Geometry check sheet. Reference: the model listing, model coordinates, mm. A direction names the side the tool comes from. Give positions to 0.01 mm unless a question says otherwise; leave off trailing zeros. Loops run counter-clockwise (first coordinate to the right, second up) from the corner with the lowest first, then second, coordinate; pieces in that order, holes last. Notation, with made-up numbers: (83.25, 25.5) - (105.25, 25.5) arc R26 ccw to (105.25, 46.5) - close; hole circle Ø10 at (18.25, -4). An arc over 180 degrees is marked (long way). Use a Markdown table: item, result. Add a question column.
1. Draft check along Y on faces 5 (the flat face through (-2, 2, -2)), 6 (the cylindrical face through (2, -5, -53)), 7 (the flat face through (-51, -10, 31)). Enter one of: pulls with the +Y half, pulls with the -Y half, needs draft (parallel to the pull), parting line crosses it, or undercut.
2. Cross-section at A-A on z = -55. Enter the section's corners in (x, y).
3. Depth check by flat-ended pin: P1, Ø1, axis at x = -61.5, y = 3.5, coming from the -Z side; P2, Ø6, axis at x = 18.5, y = 1, coming from the +Z side; P3, Ø7.5, axis at x = 3, z = -2, coming from the +Y side; P4, Ø2, axis at x = -2.5, y = -3, coming from the -Z side. Enter the tip coordinate at first touch or a pass-through.
4. Material ranges on L1, parallel to Y at x = 2.2, z = -55; L2, parallel to X at y = -8.5, z = -63.5; L3, parallel to X at y = 6.25, z = 0, recorded low to high.
5. Cross-section at B-B on z = 0. Enter the section's corners in (x, y), and give its area (3 significant figures).
6. Cross-section at C-C on y = 5.75. Enter the section's corners in (x, z).
7. Set-up check for faces 1 (the flat face through (51.29, -4.93, 30.883)), 2 (the flat face through (-1.1, -5, -60)), 3 (the flat face through (-54.171, 1.014, 33.717)), 4 (the flat face through (50.533, -4.93, 32.755)): record each of +Z, -Z, +X, -X, +Y, -Y from which the full face is reachable in a straight line by a thin tool's end or side.
8. Cross-section at D-D on z = -20.5. Enter the section's corners in (x, y), and give its area (3 significant figures).
from build123d import *

# Parameters (mm, degrees)
BOSS_EXTRUDE1_DEPTH = 2
BOSS_EXTRUDE1_DRAFT = 45
SKETCH2_R           = 2.5
CUT_EXTRUDE1_DEPTH  = 114.154761278
SKETCH3_R           = 9
SKETCH3_R_2         = 7.5
BOSS_EXTRUDE2_DEPTH = 8
SKETCH4_W           = 2
SKETCH4_H           = 20
BOSS_EXTRUDE3_DEPTH = 10
SKETCH5_R           = 2
CUT_EXTRUDE2_DEPTH  = 10
CIRPATTERN1_COUNT   = 3
CUT_EXTRUDE3_DEPTH  = 1000


# Read off the part's stored shape, not the designer's step: Boss-Extrude1
with BuildPart() as part:
    # Boss-Extrude1 outline → Boss-Extrude1 (with draft: the straight prism first)
    with BuildSketch(Plane(origin=(0, 2, 0), x_dir=(1, 0, 0), z_dir=(0, 1, 0))):
        with BuildLine():
            ThreePointArc((-3.1, 77.938373091), (-67.549981495, 39), (-69.046611026, -36.284507794))
            Line((-69.046611026, -36.284507794), (-43.119219382, -21.315321248))
            Line((-43.119219382, -21.315321248), (-40.019219382, -26.684678752))
            Line((-40.019219382, -26.684678752), (-65.946611026, -41.653865297))
            ThreePointArc((-65.946611026, -41.653865297), (0, -78), (65.946611026, -41.653865297))
            Line((65.946611026, -41.653865297), (40.019219382, -26.684678752))
            Line((40.019219382, -26.684678752), (43.119219382, -21.315321248))
            Line((43.119219382, -21.315321248), (69.046611026, -36.284507794))
            ThreePointArc((69.046611026, -36.284507794), (67.549981495, 39), (3.1, 77.938373091))
            Line((3.1, 77.938373091), (3.1, 48))
            Line((3.1, 48), (-3.1, 48))
            Line((-3.1, 48), (-3.1, 77.938373091))
        make_face()
    extrude(amount=-BOSS_EXTRUDE1_DEPTH)
    # Boss-Extrude1: the draft: its side faces are tilted about the plane it starts from
    boss_extrude1_sides = [part.faces().sort_by_distance(p)[0] for p in [
        (67.549981495, 1, -39),
        (3.1, 1, -62.969186546),
        (0, 1, -48),
        (-3.1, 1, -62.969186546),
        (-67.549981495, 1, -39),
        (-56.082915204, 1, 28.799914521),
        (-41.569219382, 1, 24),
        (-52.982915204, 1, 34.169272025),
        (0, 1, 78),
        (52.982915204, 1, 34.169272025),
        (41.569219382, 1, 24),
        (56.082915204, 1, 28.799914521),
    ]]
    draft(boss_extrude1_sides, Plane(origin=(0, 2, 0), x_dir=(1, 0, 0), z_dir=(0, 1, 0)), BOSS_EXTRUDE1_DRAFT)

    # Sketch2 → Cut-Extrude1 (cut, through all)
    with BuildSketch(Plane(origin=(0, 2, 0), x_dir=(1, 0, 0), z_dir=(0, 1, 0))):
        with Locations(Location((0, 0, 0), (0, 0, 270))):
            Circle(SKETCH2_R)
    extrude(amount=-CUT_EXTRUDE1_DEPTH, mode=Mode.SUBTRACT)

    # Sketch3 → Boss-Extrude2 (add)
    with BuildSketch(Plane(origin=(0, 2, 0), x_dir=(1, 0, 0), z_dir=(0, 1, 0))):
        with Locations(Location((0, 0, 0), (0, 0, 270))):
            Circle(SKETCH3_R)
        with Locations(Location((0, 0, 0), (0, 0, 270))):
            Circle(SKETCH3_R_2, mode=Mode.SUBTRACT)
    extrude(amount=BOSS_EXTRUDE2_DEPTH)

    # Sketch4 → Boss-Extrude3 (add)
    with BuildSketch(Plane.XZ):
        Polygon((42.751270189, 25.952627944), (60.071778265, 35.952627944), (59.071778265, 37.684678752), (41.751270189, 27.684678752), align=None)
        Polygon((43.851270189, 24.047372056), (61.171778265, 34.047372056), (62.171778265, 32.315321248), (44.851270189, 22.315321248), align=None)
        with Locations((2.1, -60)):
            Rectangle(SKETCH4_W, SKETCH4_H)
        with Locations((-2.1, -60)):
            Rectangle(SKETCH4_W, SKETCH4_H)
        Polygon((-44.851270189, 22.315321248), (-62.171778265, 32.315321248), (-61.171778265, 34.047372056), (-43.851270189, 24.047372056), align=None)
        Polygon((-42.751270189, 25.952627944), (-60.071778265, 35.952627944), (-59.071778265, 37.684678752), (-41.751270189, 27.684678752), align=None)
    extrude(amount=BOSS_EXTRUDE3_DEPTH)

    # Sketch5 → Cut-Extrude2 (cut)
    with BuildSketch(Plane(origin=(3.1, 0, 0), x_dir=(0, 0, -1), z_dir=(1, 0, 0))):
        with Locations((55, -5)):
            Circle(SKETCH5_R)
    cut_extrude2 = extrude(amount=-CUT_EXTRUDE2_DEPTH, mode=Mode.SUBTRACT)

    # CirPattern1: Cut-Extrude2 ×3 about axis
    cirpattern1_axis = Axis((0, 10, 0), (0, -1, 0))
    for i in range(1, CIRPATTERN1_COUNT):
        add(cut_extrude2.rotate(cirpattern1_axis, i * 360 / CIRPATTERN1_COUNT), mode=Mode.SUBTRACT)

    # Sketch6 → Cut-Extrude3 (cut)
    with BuildSketch(Plane(origin=(0, 2, 0), x_dir=(1, 0, 0), z_dir=(0, 1, 0))):
        with BuildLine():
            Line((20, 75.3923073), (20, 77.459666924))
            ThreePointArc((20, 77.459666924), (69.282032303, 40), (77.082039325, -21.409325386))
            Line((77.082039325, -21.409325386), (75.291653372, -20.375645574))
            Line((75.291653372, -20.375645574), (20, 11.547005384))
            Line((20, 11.547005384), (20, 75.3923073))
        make_face()
        with BuildLine():
            Line((-31.569219382, -41.320508076), (0, -23.094010768))
            Line((0, -23.094010768), (31.569219382, -41.320508076))
            Line((31.569219382, -41.320508076), (55.291653372, -55.016661726))
            Line((55.291653372, -55.016661726), (57.082039325, -56.050341538))
            ThreePointArc((57.082039325, -56.050341538), (0, -80), (-57.082039325, -56.050341538))
            Line((-57.082039325, -56.050341538), (-55.291653372, -55.016661726))
            Line((-55.291653372, -55.016661726), (-31.569219382, -41.320508076))
        make_face()
        with BuildLine():
            Line((-51.569219382, -6.679491924), (-20, 11.547005384))
            Line((-20, 11.547005384), (-20, 75.3923073))
            Line((-20, 75.3923073), (-20, 77.459666924))
            ThreePointArc((-20, 77.459666924), (-69.282032303, 40), (-77.082039325, -21.409325386))
            Line((-77.082039325, -21.409325386), (-75.291653372, -20.375645574))
            Line((-75.291653372, -20.375645574), (-51.569219382, -6.679491924))
        make_face()
    extrude(amount=-CUT_EXTRUDE3_DEPTH, mode=Mode.SUBTRACT)


solid = part.part
Values found:
| question | item | result |
|---|---|---|
| 1 | face 5 | pulls with the +Y half |
| 1 | face 6 | undercut |
| 1 | face 7 | pulls with the -Y half |
| 2 | outline | (-20, 0) - (-3.1, 0) - (-3.1, -3) - (-1.1, -3) - (-1.1, 0) - (-3.1, 2) - (-20, 2) - close; (-3.1, -10) - (-1.1, -10) - (-1.1, -7) - (-3.1, -7) - close; (1.1, -10) - (3.1, -10) - (3.1, -7) - (1.1, -7) - close; (1.1, -3) - (3.1, -3) - (3.1, 0) - (20, 0) - (20, 2) - (3.1, 2) - (1.1, 0) - close |
| 3 | P1 | passes through |
| 3 | P2 | stops at z = 35.51 |
| 3 | P3 | stops at y = 2 |
| 3 | P4 | stops at z = -70 |
| 4 | L1 | y = -10 to -7, -3 to 1.1 |
| 4 | L2 | x = -3.1 to -1.1, 1.1 to 3.1 |
| 4 | L3 | x = -9 to -7.5, 7.5 to 9 |
| 5 | outline | (-40, 0) - (-2.5, 0) - (-2.5, 2) - (-7.5, 2) - (-7.5, 10) - (-9, 10) - (-9, 2) - (-40, 2) - close; (2.5, 0) - (40, 0) - (40, 2) - (9, 2) - (9, 10) - (7.5, 10) - (7.5, 2) - (2.5, 2) - close |
| 5 | area | 174 mm2 |
| 6 | outline | circle Ø18 at (0, 0); hole circle Ø15 at (0, 0) |
| 7 | face 1 | +Y, -Y |
| 7 | face 2 | +Z, -Z, +Y, -Y |
| 7 | face 3 | +Y |
| 7 | face 4 | +Z, -Y |
| 8 | outline | (-20, 0) - (20, 0) - (20, 2) - (-20, 2) - close |
| 8 | area | 80.0 mm2 |
